Job drawing, mm, ordinate dimensions from the low corner. One solid piece. A direction names the side the tool comes from. Coordinates: 2 decimals unless noted, no trailing zeros. Loops run counter-clockwise (first coordinate to the right, second up) from the corner with the lowest first, then second, coordinate; pieces in that order, holes last. Notation, with made-up numbers: M 1.5,14 L 52.5,14 A24 cw 52.5,39 Z; hole C 66,-6 d11. An arc over 180 degrees is marked long. Answer as a JSON object with one key per item and string values. Group by question number.
1. Drill centre lines: L1, parallel to Z at x = 43, y = 30; L2, parallel to Y at x = 63.5, z = 68; L3, parallel to Z at x = 39.5, y = 80. Where is each one in solid material? Low to high.
2. Drop flat-ended pins along their axis: pin 1 Ø10 at (x, z) = (104, 45) entering from -Y; pin 2 Ø5 at (x, y) = (35, 79) entering from +Z; pin 3 Ø1.5 at (x, z) = (28.5, 84.5) entering from +Y; pin 4 Ø3 at (y, z) = (81, 54) entering from +X. Give the stop position or say it passes through.
3. Saw through at D-D on z = 78.5. Write the cut outline in (x, y), then the cut area to 3 significant figures.
4. Saw through at C-C on x = 60. Write the cut outline in (y, z), then the cut area to 4 significant figures.
5. Saw through at B-B on z = 59.5. Write the cut outline in (x, y).
6. Saw through at A-A on y = 23. Write the cut outline in (x, z), then the cut area to 3 significant figures.
7. 3-axis set-ups, long thin cutter, end or side, ignore diameter. For the marked faces 4, 5 and 6: which of +Z, -Z, +X, -X, +Y, -Y reach the whole face in a straight line?
8. Mould opens along Z. For the marked faces 1, 2 and 3 say: released by +Z, released by -Z, zero draft, split by the parting line, or undercut.
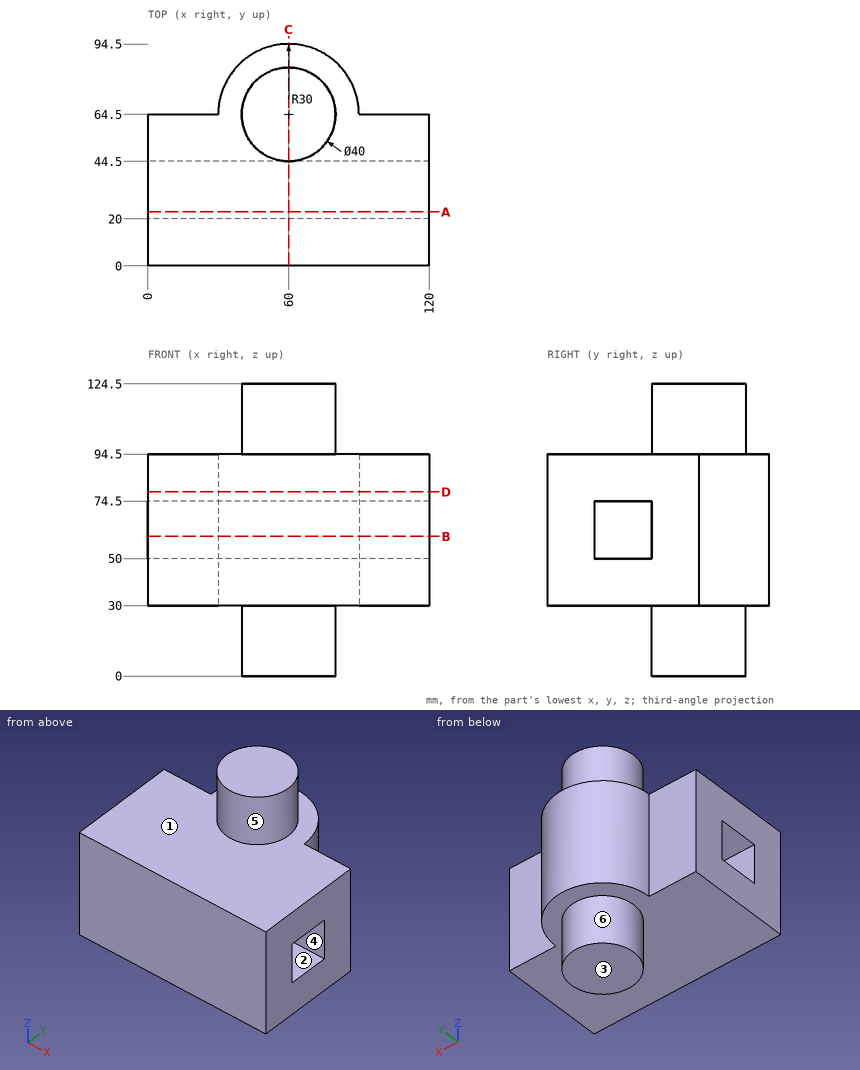
Outcome:
{
 "1": {"L1": "z = 30 to 50, 74.5 to 94.5", "L2": "y = 0 to 20, 44.5 to 94.3", "L3": "z = 30 to 94.5"},
 "2": {"pin 1": "stops at y = 0", "pin 2": "stops at z = 94.5", "pin 3": "stops at y = 64.5", "pin 4": "stops at x = 85.98"},
 "3": {"outline": "M 0,0 L 120,0 L 120,64.5 L 90,64.5 A30 ccw 30,64.5 L 0,64.5 Z", "area": "9,150 mm²"},
 "4": {"outline": "M 0,30 L 44.5,30 L 44.5,0 L 84.5,0 L 84.5,30 L 94.5,30 L 94.5,94.5 L 84.5,94.5 L 84.5,124.5 L 44.5,124.5 L 44.5,94.5 L 0,94.5 Z; hole M 20,50 L 44.5,50 L 44.5,74.5 L 20,74.5 Z", "area": "7,895 mm²"},
 "5": {"outline": "M 0,0 L 120,0 L 120,20 L 0,20 Z; M 0,44.5 L 120,44.5 L 120,64.5 L 90,64.5 A30 ccw 30,64.5 L 0,64.5 Z"},
 "6": {"outline": "M 0,30 L 120,30 L 120,50 L 0,50 Z; M 0,74.5 L 120,74.5 L 120,94.5 L 0,94.5 Z", "area": "4,800 mm²"},
 "7": {"face 4": "+X, -X", "face 5": "+Z", "face 6": "-Z"},
 "8": {"face 1": "released by +Z", "face 2": "undercut", "face 3": "released by -Z"}
}
